The listing builds one solid part. Answer for the finished solid, in the listing's coordinates (mm). A direction names the side the tool comes from. Give positions to 0.01 mm unless a question says otherwise; leave off trailing zeros. Write each loop counter-clockwise with the first axis right and the second up, starting at its lowest first coordinate (ties: lowest second). Pieces come first, ordered by that corner, then holes. Notation, with made-up numbers: (-24, 31) -> (-17, 31) arc R20 cw to (-17, 54) -> close; hole circle Ø11 at (-27.5, 22.25). An arc over 180 degrees is marked (long way). Put each result on its own line as item: value. Start each with the question number.
1) A cutting plane is placed at A-A (z = 0.8). Write down the section's boundary in (x, y).
2) For a pull along Y with two mould halves and no side action, classify faces 4 (the flat face through (0, 0, 0)), 5 (the flat face through (0, -23.749, 3)), 6 (the flat face through (2, 9.686, 4)) as released by +Y, released by -Y, zero draft, split by the parting line, or undercut.
3) A cutting plane is placed at B-B (y = 25). Write down the section's boundary in (x, z) (3 decimals).
4) Find the intervals of material crossed by line 1 along Y through (x, z) = (6.25, 4.6); line 2 along Y through (x, z) = (4, 1); line 3 along Z through (x, y) = (4.75, 3.5), in increasing order. Write a range as from..to.
5) For faces 1 (the flat face through (0, 28, 4.245)), 2 (the flat face through (-5.08, 28, 3)), 3 (the flat face through (5.287, 5.32, 4.269)), determine the directions among +Z, -Z, +X, -X, +Y, -Y from which every point of the face is accessible in a straight line to the end or side of a thin tool.
6) Flat-ended cylindrical pins translate along their axes: pin 1 Ø3 at (y, z) = (26, 3.5) entering from -X; pin 2 Ø8.5 at (x, y) = (-1, 29.5) entering from +Z (3 decimals); pin 3 Ø1.5 at (x, z) = (5.5, 5.5) entering from +Y. Find the tip coordinate at first contact, or state that the pin passes through.
from build123d import *

# Parameters (mm, degrees)
SKETCH1_W           = 17.38
SKETCH1_H           = 47.498
BOSS_EXTRUDE1_DEPTH = 5.95
CUT_EXTRUDE1_DEPTH  = 3.41
SKETCH3_W           = 10.16
SKETCH3_H           = 2.54
BOSS_EXTRUDE2_DEPTH = 7.62


with BuildPart() as part:
    # Sketch1 → Boss-Extrude1 (new body)
    with BuildSketch(Plane.XY):
        Rectangle(SKETCH1_W, SKETCH1_H)
    extrude(amount=BOSS_EXTRUDE1_DEPTH)

    # Sketch2 → Cut-Extrude1 (cut)
    with BuildSketch(Plane.XY.offset(5.95)):
        with BuildLine():
            Line((8.21521828, 9.685626239), (8.21521828, 9.211700107))
            Line((8.21521828, 9.211700107), (7.849511502, 8.640749728))
            add(Edge.make_bspline(
                [(7.849511502, 8.640749728), (7.659628318, 8.334002218), (7.295032049, 7.745013788), (6.782872216, 6.88889346), (6.32474967, 6.098434688), (5.785332579, 5.145897577), (5.201924307, 4.005544018), (4.689678821, 2.864966249), (4.323103082, 1.941121665), (4.060487027, 1.215232336), (3.79297562, 0.453893084), (3.625200839, -0.069861436), (3.539395894, -0.337724864)],
                knots=[0, 0, 0, 0, 1.083039837, 2.079553741, 2.994830702, 3.825809671, 5.365663433, 6.838340046, 7.577558492, 8.349012095, 9.155636346, 10, 10, 10, 10], degree=3))
            add(Edge.make_bspline(
                [(3.539395894, -0.337724864), (3.294518486, -1.175139297), (2.807311479, -2.84125535), (2.421476965, -4.533716864), (2.229568553, -5.375522327)],
                knots=[0, 0, 0, 0, 1.005229416, 2, 2, 2, 2], degree=3))
            add(Edge.make_bspline(
                [(2.229568553, -5.375522327), (2.14861537, -5.818843498), (1.990394666, -6.685302183), (1.890335658, -7.560371208), (1.841471563, -7.987713605)],
                knots=[0, 0, 0, 0, 1.023294424, 2, 2, 2, 2], degree=3))
            Line((1.841471563, -7.987713605), (-2.278327252, -7.987713605))
            add(Edge.make_bspline(
                [(-2.278327252, -7.987713605), (-2.228426027, -7.742123959), (-2.132197133, -7.268531969), (-1.955335735, -6.592737484), (-1.766303583, -5.973619712), (-1.61053551, -5.589751553), (-1.535718589, -5.405375942)],
                knots=[0, 0, 0, 0, 1.116992291, 2.153993903, 3.113345314, 4, 4, 4, 4], degree=3))
            add(Edge.make_bspline(
                [(-1.535718589, -5.405375942), (-1.432470379, -5.170955855), (-1.233678754, -4.719609045), (-0.927100645, -4.077764225), (-0.630798746, -3.494030209), (-0.424952864, -3.130831897), (-0.326647197, -2.957379545)],
                knots=[0, 0, 0, 0, 1.125146569, 2.166330209, 3.124295659, 4, 4, 4, 4], degree=3))
            add(Edge.make_bspline(
                [(-0.326647197, -2.957379545), (-0.160956821, -2.676902535), (0.175753632, -2.106926516), (0.708141987, -1.248784349), (1.266217599, -0.367355885), (1.86140604, 0.532183687), (2.487318367, 1.452627488), (3.145855822, 2.393106788), (3.830525284, 3.357049593), (4.305847593, 4.000507598), (4.546955386, 4.326902418)],
                knots=[0, 0, 0, 0, 0.891601375, 1.811882565, 2.763935491, 3.74693406, 4.763958923, 5.810457796, 6.889352178, 8, 8, 8, 8], degree=3))
            Line((4.546955386, 4.326902418), (6.04709952, 6.342021403))
            Line((6.04709952, 6.342021403), (-1.737230487, 6.342021403))
            add(Edge.make_bspline(
                [(-1.737230487, 6.342021403), (-1.941407392, 6.33928709), (-2.324644322, 6.334154827), (-2.863158098, 6.274892972), (-3.328967641, 6.178379532), (-3.727025146, 6.035733564), (-4.070606045, 5.846274621), (-4.356427977, 5.588671706), (-4.60409946, 5.276798523), (-4.806692036, 4.896670937), (-4.974895269, 4.437516142), (-5.119721138, 3.888492313), (-5.250293202, 3.239224301), (-5.314926889, 2.771224888), (-5.349517854, 2.520758735)],
                knots=[0, 0, 0, 0, 1.211762192, 2.274459111, 3.211702032, 4.029445416, 4.776937485, 5.525195333, 6.297980953, 7.13082587, 8.070422764, 9.195545804, 10.499098859, 12, 12, 12, 12], degree=3))
            Line((-5.349517854, 2.520758735), (-5.827175687, 2.520758735))
            Line((-5.827175687, 2.520758735), (-4.935298951, 9.685626239))
            Line((-4.935298951, 9.685626239), (8.21521828, 9.685626239))
        make_face()
    extrude(amount=-CUT_EXTRUDE1_DEPTH, mode=Mode.SUBTRACT)

    # Sketch3 → Boss-Extrude2 (add)
    with BuildSketch(Plane(origin=(0, 23.749, 0), x_dir=(1, 0, 0), z_dir=(0, 1, 0))):
        with Locations((0, -2.975)):
            Rectangle(SKETCH3_W, SKETCH3_H)
    extrude(amount=BOSS_EXTRUDE2_DEPTH)


solid = part.part
Reply:
1. outline: (-8.69, -23.75) -> (8.69, -23.75) -> (8.69, 23.75) -> (-8.69, 23.75) -> close
2. face 4: zero draft
2. face 5: released by -Y
2. face 6: undercut
3. outline: (-5.08, 1.705) -> (5.08, 1.705) -> (5.08, 4.245) -> (-5.08, 4.245) -> close
4. line 1: y = -23.75..5.96, 9.69..23.75
4. line 2: y = -23.75..23.75
4. line 3: z = 0..2.54
5. face 1: +Z, +X, -X, +Y
5. face 2: +Z, -Z, -X, +Y
5. face 3: +Z
6. pin 1: stops at x = -5.08
6. pin 2: stops at z = 4.245
6. pin 3: stops at y = 23.75
